Model file for the job. Use its own axes, mm. Face numbers are marked on the shaded views. A direction names the side the tool comes from. Round coordinates to 2 decimals unless told otherwise and drop trailing zeros. Write each loop counter-clockwise with the first axis right and the second up, starting at its lowest first coordinate (ties: lowest second). Pieces come first, ordered by that corner, then holes. Notation, with made-up numbers: (32.25, -6.5) - (91.25, -6.5) arc R14 ccw to (91.25, 5.5) - close; hole circle Ø11 at (63.5, -6). An arc over 180 degrees is marked (long way). One line per item, written item: value.
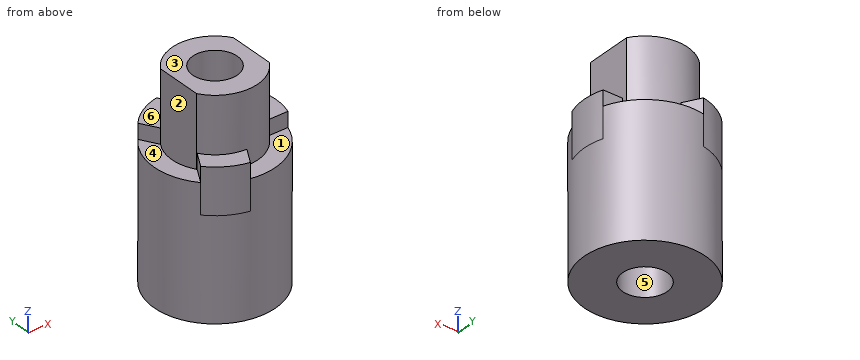
from build123d import *

# Parameters (mm, degrees)
SKETCH_R      = 6
PAD_DEPTH     = 10
PAD001_DEPTH  = 10
SKETCH002_R   = 2.2
POCKET_DEPTH  = 20.001
PAD002_DEPTH  = 4.5
SKETCH004_R   = 6
SKETCH004_R_2 = 4.25
PAD003_DEPTH  = 3


with BuildPart() as part:
    # Sketch → Pad (new body)
    with BuildSketch(Plane.XY):
        Circle(SKETCH_R)
    extrude(amount=PAD_DEPTH)

    # Sketch001 (on Face3 of Pad) → Pad001 (join)
    with BuildSketch(Plane.XY.offset(10)):
        with BuildLine():
            ThreePointArc((-3.6, -2.258871), (0, -4.25), (3.6, -2.258871))
            Line((3.6, -2.258871), (3.6, 2.258871))
            ThreePointArc((3.6, 2.258871), (0, 4.25), (-3.6, 2.258871))
            Line((-3.6, -2.258871), (-3.6, 2.258871))
        make_face()
    extrude(amount=PAD001_DEPTH)

    # Sketch002 (on Face8 of Pad001) → Pocket (cut, through all)
    with BuildSketch(Plane.XY.offset(20)):
        Circle(SKETCH002_R)
    extrude(amount=-POCKET_DEPTH, mode=Mode.SUBTRACT)

    # Sketch003 (on Face3 of Pocket) → Pad002 (join)
    with BuildSketch(Plane.XY.offset(10)):
        with BuildLine():
            ThreePointArc((3.776242, -1.95), (4.25, 0), (3.776242, 1.95))
            Line((3.776242, 1.95), (5.674284, 1.95))
            ThreePointArc((5.674284, -1.95), (6, 0), (5.674284, 1.95))
            Line((3.776242, -1.95), (5.674284, -1.95))
        make_face()
        with BuildLine():
            ThreePointArc((-1.148393, 5.889074), (-3, 5.196152), (-4.525892, 3.939074))
            Line((-3.57687, 2.295321), (-4.525892, 3.939074))
            ThreePointArc((-0.199371, 4.245321), (-2.125, 3.680608), (-3.57687, 2.295321))
            Line((-1.148393, 5.889074), (-0.199371, 4.245321))
        make_face()
        with BuildLine():
            ThreePointArc((-4.525892, -3.939074), (-3, -5.196152), (-1.148393, -5.889074))
            Line((-1.148393, -5.889074), (-0.199371, -4.245321))
            ThreePointArc((-3.57687, -2.295321), (-2.125, -3.680608), (-0.199371, -4.245321))
            Line((-4.525892, -3.939074), (-3.57687, -2.295321))
        make_face()
    extrude(amount=PAD002_DEPTH)

    # Sketch004 (on Face4 of Pad002) → Pad003 (join)
    with BuildSketch(Plane.XY.offset(10)):
        Circle(SKETCH004_R)
        Circle(SKETCH004_R_2, mode=Mode.SUBTRACT)
    extrude(amount=PAD003_DEPTH)


solid = part.part
1. Band-saw the part on A-A on z = 14. Write the cut outline in (x, y).
Report:
outline: (-4.53, -3.94) arc R6 ccw to (-1.15, -5.89) - (-0.2, -4.25) arc R4.25 ccw to (3.6, -2.26) - (3.6, 2.26) arc R4.25 ccw to (-0.2, 4.25) - (-1.15, 5.89) arc R6 ccw to (-4.53, 3.94) - (-3.58, 2.3) arc R4.25 ccw to (-3.6, 2.26) - (-3.6, -2.26) arc R4.25 ccw to (-3.58, -2.3) - close; (3.78, -1.95) - (5.67, -1.95) arc R6 ccw to (5.67, 1.95) - (3.78, 1.95) arc R4.25 cw to start; hole circle Ø4.4 at (0, 0)
2. Band-saw the part on B-B on y = 0. Write the cut outline in (x, z).
Report:
outline: (-6, 0) - (-2.2, 0) - (-2.2, 20) - (-3.6, 20) - (-3.6, 10) - (-4.25, 10) - (-4.25, 13) - (-6, 13) - close; (2.2, 0) - (6, 0) - (6, 14.5) - (4.25, 14.5) - (4.25, 10) - (3.6, 10) - (3.6, 20) - (2.2, 20) - close
3. Drop flat-ended pins along their axis: pin 1 (1.5 mm diameter, centred on x = -1.5, z = 15.5, fed in from +Y); pin 2 (0.7 mm diameter, centred on x = 5, y = 1, fed in from +Z); pin 3 (1.6 mm diameter, centred on x = 4.5, z = 14, fed in from -Y). Give the stop position or say it passes through.
Report:
pin 1: y = 4.18
pin 2: z = 14.5
pin 3: y = -1.95
4. Band-saw the part on C-C on x = 1.75. Write the cut outline in (y, z).
Report:
outline: (-5.74, 0) - (-1.33, 0) - (-1.33, 20) - (-3.87, 20) - (-3.87, 13) - (-5.74, 13) - close; (1.33, 0) - (5.74, 0) - (5.74, 13) - (3.87, 13) - (3.87, 20) - (1.33, 20) - close
5. Band-saw the part on D-D on y = -1.5. Write the cut outline in (x, z), plus the area to 3 significant figures.
Report:
outline: (-5.81, 0) - (-1.61, 0) - (-1.61, 20) - (-3.6, 20) - (-3.6, 10) - (-3.98, 10) - (-3.98, 13) - (-5.81, 13) - close; (1.61, 0) - (5.81, 0) - (5.81, 14.5) - (3.98, 14.5) - (3.98, 10) - (3.6, 10) - (3.6, 20) - (1.61, 20) - close
area: 138 mm²
6. Mould opens along Y. For the marked faces 4, 5 and 6 say: released by +Y, released by -Y, zero draft, split by the parting line, or undercut.
Report:
face 4: undercut
face 5: undercut
face 6: zero draft
7. Tool access for the marked faces 1, 2 and 3: list every direction of +Z, -Z, +X, -X, +Y, -Y with a clear straight run to the whole face (end or side of a thin tool).
Report:
face 1: +Z, +X, -Y
face 2: +Z
face 3: +Z, +X, -X, +Y, -Y
8. Wall check: probe 1 along Y at (x, z) = (0, 5); probe 2 along X at (y, z) = (0.5, 11.75); probe 3 along Y at (x, z) = (1.75, 1). Give the ranges that are in metal, low to high. Write a range as [from, to].
Report:
probe 1: [-6, -2.2], [2.2, 6]
probe 2: [-5.98, -4.22], [-3.6, -2.14], [2.14, 3.6], [4.22, 5.98]
probe 3: [-5.74, -1.33], [1.33, 5.74]
